Autodesk Inventor part; units mm, degrees
ref_plane "YZ Plane" through (0, 0, 0) normal (1, 0, 0) x (0, 1, 0)
ref_plane "XZ Plane" through (0, 0, 0) normal (0, 1, 0) x (-1, 0, 0)
ref_plane "XY Plane" through (0, 0, 0) normal (0, 0, 1) x (1, 0, 0)
sketch "Sketch1" plane through (0, 0, 0) normal (0, 0, 1) x (1, 0, 0)
  line L0 (-13.1198, 5.618) -> (5.8802, 5.618)
  line L1 (5.8802, 5.618) -> (5.8802, -13.382)
  line L2 (5.8802, -13.382) -> (-13.1198, -13.382)
  line L3 (-13.1198, -13.382) -> (-13.1198, 5.618)
  point P0 (0, 0)
  dimension "d0" = 19
  dimension "d1" = 19
extrude "Extrusion1" add sketch "Sketch1" along normal blind 7
sketch "Sketch2" plane through (0, 0, 7) normal (0, 0, 1) x (1, 0, 0)
  line L0 (5.8802, 5.618) -> (-13.1198, 5.618)
  line L1 (-13.1198, 5.618) -> (-13.1198, -13.382)
  line L2 (-13.1198, -13.382) -> (5.8802, -13.382)
  line L3 (5.8802, -13.382) -> (5.8802, 5.618)
  line L4 (-13.1198, -13.382) -> (5.8802, -13.382)
  line L5 (-8.1198, -13.382) -> (-8.1198, 5.618)
  line L6 (5.8802, 5.618) -> (-13.1198, 5.618)
  line L7 (0.8802, -13.382) -> (0.8802, 5.618)
  line L8 (-13.1198, 3.1934) -> (-8.1198, 3.1934) construction
  line L9 (-8.1198, 3.1934) -> (0.8802, 3.1934) construction
  line L10 (0.8802, 3.1934) -> (5.8802, 3.1934) construction
  point P0 (0, 0)
  dimension "d4" = 9
extrude "Extrusion2" add sketch "Sketch2" along normal blind 15 contours L3 L2 L7 L0 | L5 L2 L1 L0
sketch "Sketch3" plane through (0, 0, 0) normal (0, 0, -1) x (-1, 0, 0)
  circle A0 centre (3.6198, -3.882) radius 2.125
  line L0 (13.1198, 5.618) -> (-5.8802, 5.618)
  line L1 (13.1198, -13.382) -> (8.1198, -13.382)
  line L2 (-5.8802, 5.618) -> (13.1198, -13.382) construction
  line L3 (13.1198, 5.618) -> (-5.8802, -13.382) construction
  point P0 (0, 0)
  dimension "d7" = 4.25
extrude "Extrusion3" cut sketch "Sketch3" against normal up to next
sketch "Sketch4" plane through (5.8802, -13.382, 0) normal (1, 0, 0) x (0, 0, -1)
  circle A0 centre (-14.5, 9.5) radius 1.575
  line L0 (-7, 0) -> (-7, 19)
  line L1 (-7, 0) -> (-22, 0)
  line L2 (-22, 0) -> (-7, 19) construction
  line L3 (-22, 0) -> (-22, 19)
  line L4 (-7, 0) -> (-22, 19) construction
  point P0 (0, 13.382)
  dimension "d10" = 3.15
extrude "Extrusion4" cut sketch "Sketch4" against normal through all
sketch "Sketch5" plane through (0, 0, 7) normal (0, 0, 1) x (1, 0, 0)
  line L0 (-3.6198, 0.243) -> (-0.0475, -1.8195)
  line L1 (-0.0475, -1.8195) -> (-0.0475, -5.9445)
  line L2 (-0.0475, -5.9445) -> (-3.6198, -8.007)
  line L3 (-3.6198, -8.007) -> (-7.1922, -5.9445)
  line L4 (-7.1922, -5.9445) -> (-7.1922, -1.8195)
  line L5 (-7.1922, -1.8195) -> (-3.6198, 0.243)
  circle A0 centre (-3.6198, -3.882) radius 2.125
  point P0 (0, 0)
  dimension "d13" = 8.25
extrude "Extrusion5" cut sketch "Sketch5" against normal blind 3.2
properties part number "YPulleySupportHolder"
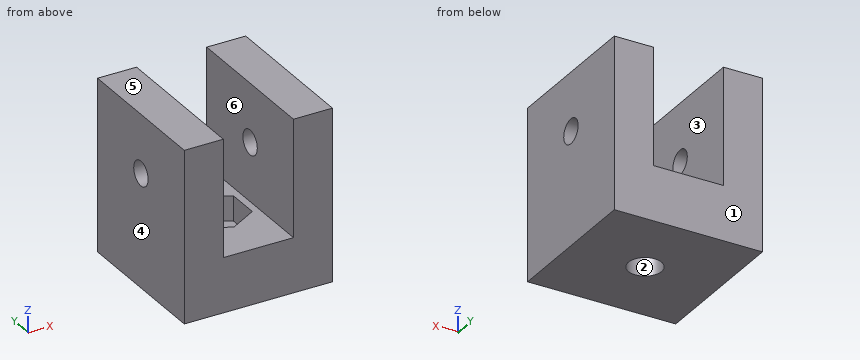
Here's how the part is built. I have some questions about the finished solid (model axes, mm). Face numbers are marked on the shaded views. A direction names the side the tool comes from. Coordinates: 2 decimals unless noted, no trailing zeros. Write each loop counter-clockwise with the first axis right and the second up, starting at its lowest first coordinate (ties: lowest second). Pieces come first, ordered by that corner, then holes.
Item 1: I want a section at C-C on z = 20.25. Write out the boundary of the cut face in (x, y), and give its area (3 significant figures).
Item 2: If I drill on line 1 (X direction, y = -2, z = 10); line 2 (Y direction, x = -10, z = 14.5); line 3 (Y direction, x = -12, z = 14.25), over which ranges is the centre line in solid material (lowest first)?
Item 3: I want a section at D-D on x = -4. Write out the boundary of the cut face in (y, z), and give its area (3 significant figures).
Item 4: If we mould it in two halves opening along X, with no side actions, what happens to the marked faces 1, 2, 3 and 4? For each: +X half, -X half, draft (parallel to the pull), parting line (faces both ways), or undercut.
Item 5: On a 3-axis mill with a long thin cutter (end or side, diameter ignored), from which of +Z, -Z, +X, -X, +Y, -Y can I reach the whole of each face in a straight line? I mean the marked faces 5 and 6. Say none if no direction works.
Item 6: I want a section at B-B on z = 5.5. Write out the boundary of the cut face in (x, y), and give its area (3 significant figures).
Item 7: Will these pins go through, and if not, where does the flat tip stop? pin 1 (1.5 mm diameter, centred on x = -1, z = 11, fed in from +Y); pin 2 (3.5 mm diameter, centred on x = -5, y = -3, fed in from +Z).
Item 8: I want a section at A-A on z = 14.5. Write out the boundary of the cut face in (x, y), and give its area (4 significant figures).
Findings below:
1. outline: (-13.12, -13.38) - (-8.12, -13.38) - (-8.12, 5.62) - (-13.12, 5.62) - close; (0.88, -13.38) - (5.88, -13.38) - (5.88, 5.62) - (0.88, 5.62) - close
1. area: 190 mm2
2. line 1: x = -13.12 to -8.12, 0.88 to 5.88
2. line 2: y = -13.38 to -5.46, -2.31 to 5.62
2. line 3: y = -13.38 to -5.44, -2.33 to 5.62
3. outline: (-13.38, 0) - (-5.97, 0) - (-5.97, 3.8) - (-7.79, 3.8) - (-7.79, 7) - (-13.38, 7) - close; (-1.79, 0) - (5.62, 0) - (5.62, 7) - (0.02, 7) - (0.02, 3.8) - (-1.79, 3.8) - close
3. area: 92.1 mm2
4. face 1: draft
4. face 2: undercut
4. face 3: undercut
4. face 4: -X half
5. face 5: +Z, +X, -X, +Y, -Y
5. face 6: +Z, +Y, -Y
6. outline: (-13.12, -13.38) - (5.88, -13.38) - (5.88, 5.62) - (-13.12, 5.62) - close; hole (-7.19, -5.94) - (-3.62, -8.01) - (-0.05, -5.94) - (-0.05, -1.82) - (-3.62, 0.24) - (-7.19, -1.82) - close
6. area: 317 mm2
7. pin 1: passes through
7. pin 2: stops at z = 3.8
8. outline: (-13.12, -13.38) - (-8.12, -13.38) - (-8.12, -5.46) - (-13.12, -5.46) - close; (-13.12, -2.31) - (-8.12, -2.31) - (-8.12, 5.62) - (-13.12, 5.62) - close; (0.88, -13.38) - (5.88, -13.38) - (5.88, -5.46) - (0.88, -5.46) - close; (0.88, -2.31) - (5.88, -2.31) - (5.88, 5.62) - (0.88, 5.62) - close
8. area: 158.5 mm2
